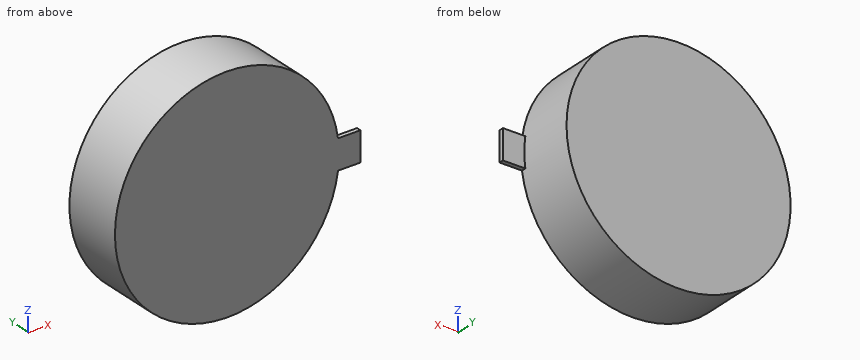
```python
from build123d import *

# Parameters (mm, degrees)
SKETCH1_R           = 5
BOSS_EXTRUDE1_DEPTH = 2.7
SKETCH2_W           = 1
SKETCH2_H           = 1.31363251
BOSS_EXTRUDE2_DEPTH = 0.2


with BuildPart() as part:
    # Sketch1 → Boss-Extrude1 (new body)
    with BuildSketch(Plane(origin=(0, 0, 0), x_dir=(1, 0, 0), z_dir=(0, 1, 0))):
        Circle(SKETCH1_R)
    extrude(amount=BOSS_EXTRUDE1_DEPTH)

    # Sketch2 → Boss-Extrude2 (add)
    with BuildSketch(Plane(origin=(0, 0, 0), x_dir=(1, 0, 0), z_dir=(0, 1, 0))):
        with Locations((5.456671505, 0)):
            Rectangle(SKETCH2_W, SKETCH2_H)
    extrude(amount=BOSS_EXTRUDE2_DEPTH)


solid = part.part
```
Input: part model. Units: mm. Frame: model coordinates. Round coordinates to 2 decimals unless told otherwise and drop trailing zeros. Loops run counter-clockwise (first coordinate to the right, second up) from the corner with the lowest first, then second, coordinate; pieces in that order, holes last. Notation, with made-up numbers: M 6,1 L 37,1 A14 ccw 37,10 Z; hole C 31,1.25 d6. An arc over 180 degrees is marked long. Answer in a Markdown table with one row per item. Add a question column.
1. Contact query for a flat-ended pin moving along its axis: pin 1 (2 mm diameter, centred on x = 0.5, z = -3, fed in from -Y). Output: stop coordinate, or through.
2. Ray query, probe 1 along X at (y, z) = (1.1, 0); probe 2 along X at (y, z) = (1.1, -2.5); probe 3 along Z at (x, y) = (-1, 2.5). Return the intervals inside material, ascending.
3. Section C-C (y = 1.9). Output: boundary loops of the cut face in (x, z), and give its area (3 significant figures).
4. Section A-A (z = 0). Output: boundary loops of the cut face in (x, y).
5. Section D-D (z = -1). Output: boundary loops of the cut face in (x, y), and give its area (3 significant figures).
6. Section B-B (x = -3). Output: boundary loops of the cut face in (y, z).
Values follow:
| question | item | result |
|---|---|---|
| 1 | pin 1 | y = 0 |
| 2 | probe 1 | -5 to 5 |
| 2 | probe 2 | -4.33 to 4.33 |
| 2 | probe 3 | -4.9 to 4.9 |
| 3 | outline | C 0,0 d10 |
| 3 | area | 78.5 mm^2 |
| 4 | outline | M -5,0 L 5.96,0 L 5.96,0.2 L 5,0.2 L 5,2.7 L -5,2.7 Z |
| 5 | outline | M -4.9,0 L 4.9,0 L 4.9,2.7 L -4.9,2.7 Z |
| 5 | area | 26.5 mm^2 |
| 6 | outline | M 0,-4 L 2.7,-4 L 2.7,4 L 0,4 Z |
